Read the model definition and answer for the solid it produces. Units are mm, in the model's axes. A direction names the side the tool comes from. Give positions to 0.01 mm unless a question says otherwise; leave off trailing zeros. Loops run counter-clockwise (first coordinate to the right, second up) from the corner with the lowest first, then second, coordinate; pieces in that order, holes last.
(1) Which of the six approach directions +Z, -Z, +X, -X, +Y, -Y give full straight-line access (tool end or side, diameter ignored) to faces 5 (the face through (-17.824, 35.009, 7.395)), 6 (the face through (-2, 18.1, 6)), 7 (the face through (-2.5, 26.1, 7.4))?
(2) Find section B-B, the plane x = -42.5. Write down the section's boundary in (y, z), then the cut area to 3 significant figures.
(3) Find section A-A, the plane z = 7.5. State how many separate pieces and enclosed holes the cut face has, then the cut area to 3 significant figures.
(4) Find section C-C, the plane x = -5. Write down the section's boundary in (y, z), then the cut area to 3 significant figures.
(5) Straight lines are drawn through the part: probe 1 along Y at (x, z) = (-34, 8.25); probe 2 along Y at (x, z) = (-2.5, 7); probe 3 along X at (y, z) = (26.7, 7.5). For each, find the intervals that lie inside material, in ascending order.
(6) Find section D-D, the plane y = 20. Write down the section's boundary in (x, z), then the cut area to 3 significant figures.
(7) Determine the mould class of faces 1 (the face through (-6.196, 24, 7)), 2 (the face through (0.088, 27.621, 5.502)), 3 (the face through (0.088, 19.621, 5.502)), 4 (the face through (-50.94, 47.23, 14.29)) for opening direction X: pulls with the +X half, pulls with the -X half, needs draft (parallel to the pull), parting line crosses it, or undercut.
(8) Each of these flat-tipped pins is pushed along its axis until it touches: P1, Ø5, axis at x = -14.5, z = 7.5, coming from the +Y side; P2, Ø4, axis at x = 0, z = 5.5, coming from the +Y side; P3, Ø1.5, axis at y = 14, z = 5, coming from the -X side; P4, Ø2.5, axis at x = -46.7, z = 7.5, coming from the -Y side. Where does it stop, or does it pass through?
```python
from build123d import *

# Parameters (mm, degrees)
EXTRUDE_1_DEPTH     = 15
CUT_EXTRUDE_1_REACH = 74.926
SKETCH_2_R          = 2
SKETCH_3_R          = 7.5
EXTRUDE_2_DEPTH     = 3
EXTRUDE_START       = -3
SKETCH_4_R          = 7.5
EXTRUDE_3_DEPTH     = 3
SKETCH_5_R          = 2
CUT_EXTRUDE_2_DEPTH = 11
FILLET_1_R          = 2.5


with BuildPart() as part:
    # 草圖1 → 填料-伸長1 (new body)
    with BuildSketch(Plane.XY):
        Polygon((-26.696480976, 45.2), (-47.696480976, 45.2), (-51.696480976, 45.2), (-51.696480976, 49.2), (-24.875445442, 49.2), (-7.375445442, 29.1), (0, 29.1), (0, 26.1), (-6.196480976, 26.1), (-6.196480976, 21.1), (0, 21.1), (0, 18.1), (-7.5, 18.1), (-25, 0), (-51.696480976, 0), (-51.696480976, 4), (-47.696480976, 4), (-26.696480976, 4), (-9.196480976, 22.1), (-9.196480976, 25.1), align=None)
    extrude(amount=EXTRUDE_1_DEPTH)

    # 除料-伸長1: up to this face of the body (flat: up to its plane)
    cut_extrude_1_end = Plane(part.part.faces().sort_by_distance((-38.285963209, 49.2, 7.5))[0])
    # 草圖2 → 除料-伸長1 (cut, up to the picked face)
    with BuildSketch(Plane.XZ, mode=Mode.PRIVATE) as cut_extrude_1_sk1:
        with Locations((-46.696480976, 7.5)):
            Circle(SKETCH_2_R)
    cut_extrude_1_tool1 = split(extrude(cut_extrude_1_sk1.sketch, amount=-CUT_EXTRUDE_1_REACH, mode=Mode.PRIVATE), bisect_by=cut_extrude_1_end, keep=Keep.BOTH, mode=Mode.PRIVATE)
    add(cut_extrude_1_tool1.solids().sort_by(Axis((-46.696481, 0, 7.5), (0, 1, 0)))[0], mode=Mode.SUBTRACT)

    # 草圖3 → 填料-伸長2 (add)
    with BuildSketch(Plane.XZ.offset(-18.1)):
        with Locations((0, 7.5)):
            Circle(SKETCH_3_R)
    extrude(amount=-EXTRUDE_2_DEPTH)

    # 草圖4 → 填料-伸長3 (add)
    with BuildSketch(Plane(origin=(0, 29.1, 0), x_dir=(1, 0, 0), z_dir=(0, 1, 0)).offset(EXTRUDE_START)):
        with Locations((0, -7.5)):
            Circle(SKETCH_4_R)
    extrude(amount=EXTRUDE_3_DEPTH)

    # 草圖5 → 除料-伸長2 (cut)
    with BuildSketch(Plane(origin=(0, 29.1, 0), x_dir=(1, 0, 0), z_dir=(0, 1, 0))):
        with Locations(Location((0, -7.5, 0), (0, 0, 270))):
            Circle(SKETCH_5_R)
    extrude(amount=-CUT_EXTRUDE_2_DEPTH, mode=Mode.SUBTRACT)

    # 圓角1
    fillet_1_edges = [part.edges().sort_by_distance(p)[0] for p in [
        (-51.696480976, 47.2, 0),
        (-51.696480976, 2, 15),
        (-51.696480976, 2, 0),
        (-51.696480976, 47.2, 15),
    ]]
    fillet(fillet_1_edges, radius=FILLET_1_R)


solid = part.part
```
Entries:
1. face 5: +Z, -Z, -X
1. face 6: +Z, -Z, +X, -Y
1. face 7: +Z, -Z, +X
2. outline: (0, 0) - (4, 0) - (4, 15) - (0, 15) - close; (45.2, 0) - (49.2, 0) - (49.2, 15) - (45.2, 15) - close
2. area: 120 mm2
3. separate pieces: 5
3. enclosed holes: 0
3. area: 466 mm2
4. outline: (18.1, 0) - (21.1, 0) - (21.1, 15) - (18.1, 15) - close; (26.1, 0) - (29.1, 0) - (29.1, 15) - (26.1, 15) - close
4. area: 90.0 mm2
5. probe 1: y = 0 to 4, 45.2 to 49.2
5. probe 2: y = 18.1 to 21.1, 26.1 to 29.1
5. probe 3: x = -10.59 to -2, 2 to 7.5
6. outline: (-11.23, 0) - (0, 0) arc R7.5 ccw to (0, 15) - (-11.23, 15) - close; hole circle Ø4 at (0, 7.5)
6. area: 244 mm2
7. face 1: pulls with the +X half
7. face 2: undercut
7. face 3: undercut
7. face 4: pulls with the -X half
8. P1: stops at y = 40.15
8. P2: stops at y = 29.1
8. P3: stops at x = -17.75
8. P4: passes through
